```python
from build123d import *

# Parameters (mm, degrees)
SKETCH1_W                                       = 100
SKETCH1_H                                       = 55
BOSS_EXTRUDE1_DEPTH                             = 5
SKETCH2_W                                       = 5
SKETCH2_H                                       = 55
BOSS_EXTRUDE2_DEPTH                             = 15
CUT_EXTRUDE1_REACH                              = 22
CSK_FOR_M2_FLAT_HEAD_MACHINE_SCREW1_D           = 2.4
CSK_FOR_M2_FLAT_HEAD_MACHINE_SCREW1_CSINK_D     = 4.4
CSK_FOR_M2_FLAT_HEAD_MACHINE_SCREW1_CSINK_ANGLE = 90
CUT_EXTRUDE2_REACH                              = 22
SKETCH6_R                                       = 4


with BuildPart() as part:
    # Sketch1 → Boss-Extrude1 (new body)
    with BuildSketch(Plane(origin=(0, 0, 0), x_dir=(0, 0, -1), z_dir=(1, 0, 0))):
        Rectangle(SKETCH1_W, SKETCH1_H)
    extrude(amount=BOSS_EXTRUDE1_DEPTH)

    # Sketch2 → Boss-Extrude2 (add)
    with BuildSketch(Plane(origin=(5, 0, 0), x_dir=(0, 0, -1), z_dir=(1, 0, 0))):
        with Locations((47.5, 0)):
            Rectangle(SKETCH2_W, SKETCH2_H)
    extrude(amount=BOSS_EXTRUDE2_DEPTH)

    # Sketch3 → Cut-Extrude1 (cut, up to next)
    with BuildSketch(Plane.ZY, mode=Mode.PRIVATE) as cut_extrude1_sk1:
        Polygon((50, 27.5), (40, 27.5), (50, 17.5), align=None)
    cut_extrude1_tool1 = extrude(cut_extrude1_sk1.sketch, amount=-CUT_EXTRUDE1_REACH, mode=Mode.PRIVATE) & part.part
    add(cut_extrude1_tool1.solids().sort_by_distance((0, 24.166667, 46.666667))[0], mode=Mode.SUBTRACT)
    # Sketch3 → Cut-Extrude1 (cut, up to next)
    with BuildSketch(Plane.ZY, mode=Mode.PRIVATE) as cut_extrude1_sk2:
        Polygon((50, -27.5), (40, -27.5), (50, -17.5), align=None)
    cut_extrude1_tool2 = extrude(cut_extrude1_sk2.sketch, amount=-CUT_EXTRUDE1_REACH, mode=Mode.PRIVATE) & part.part
    add(cut_extrude1_tool2.solids().sort_by_distance((0, -24.166667, 46.666667))[0], mode=Mode.SUBTRACT)

    # CSK for M2 Flat Head Machine Screw1 (through all)
    with Locations(Plane.XY.offset(-45)):
        with Locations((12.5, 15.5), (12.5, -15.5)):
            CounterSinkHole(CSK_FOR_M2_FLAT_HEAD_MACHINE_SCREW1_D / 2, CSK_FOR_M2_FLAT_HEAD_MACHINE_SCREW1_CSINK_D / 2, counter_sink_angle=CSK_FOR_M2_FLAT_HEAD_MACHINE_SCREW1_CSINK_ANGLE)

    # Sketch6 → Cut-Extrude2 (cut, up to next)
    with BuildSketch(Plane.ZY, mode=Mode.PRIVATE) as cut_extrude2_sk1:
        with Locations((22.5, 0)):
            Circle(SKETCH6_R)
    cut_extrude2_tool1 = extrude(cut_extrude2_sk1.sketch, amount=-CUT_EXTRUDE2_REACH, mode=Mode.PRIVATE) & part.part
    add(cut_extrude2_tool1.solids().sort_by_distance((0, 0, 22.5))[0], mode=Mode.SUBTRACT)


solid = part.part
```
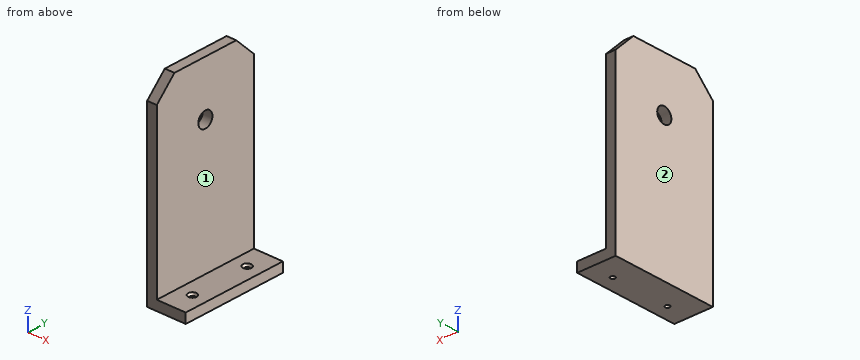
Geometry check sheet. Reference: the model listing, model coordinates, mm. Face numbers are marked on the shaded views. A direction names the side the tool comes from. Coordinates: 2 decimals unless noted, no trailing zeros. Order: outer loops, then holes, each group sorted by start corner. A loop starts at its lowest first (then second) coordinate and runs counter-clockwise, first axis right, second up.
Q1. Sectioned sample at C-C on z = 22.5. Record the cut outline in (x, y).
Reply:
outline: (0, -27.5) - (5, -27.5) - (5, -4) - (0, -4) - close; (0, 4) - (5, 4) - (5, 27.5) - (0, 27.5) - close
Q2. Sectioned sample at B-B on x = 12.5. Record the cut outline in (y, z), and give its area (3 significant figures).
Reply:
outline: (-27.5, -50) - (-16.7, -50) - (-16.7, -46) - (-17.7, -45) - (-27.5, -45) - close; (-14.3, -50) - (14.3, -50) - (14.3, -46) - (13.3, -45) - (-13.3, -45) - (-14.3, -46) - close; (16.7, -50) - (27.5, -50) - (27.5, -45) - (17.7, -45) - (16.7, -46) - close
area: 249 mm2
Q3. Thickness scan on probe 1 along Y at (x, z) = (12.5, -47); probe 2 along X at (y, z) = (-16, 9.5); probe 3 along Z at (x, y) = (14, -23.5). Record the ranges inside material, lowest first.
Reply:
probe 1: y = -27.5 to -16.7, -14.3 to 14.3, 16.7 to 27.5
probe 2: x = 0 to 5
probe 3: z = -50 to -45
Q4. Depth check by flat-ended pin: pin 1 Ø8 at (y, z) = (6.5, -25) entering from +X; pin 2 Ø6.5 at (y, z) = (0, 22.5) entering from +X; pin 3 Ø3 at (x, y) = (12.5, 15.5) entering from +Z; pin 4 Ø2 at (x, y) = (11, -12) entering from +Z. Enter the tip coordinate at first touch or a pass-through.
Reply:
pin 1: stops at x = 5
pin 2: passes through
pin 3: stops at z = -45.7
pin 4: stops at z = -45
Q5. Sectioned sample at D-D on y = -8.5. Record the cut outline in (x, z), and give its area (3 significant figures).
Reply:
outline: (0, -50) - (20, -50) - (20, -45) - (5, -45) - (5, 50) - (0, 50) - close
area: 575 mm2
Q6. Sectioned sample at A-A on y = -15.5. Record the cut outline in (x, z), and give its area (3 significant figures).
Reply:
outline: (0, -50) - (11.3, -50) - (11.3, -46) - (10.3, -45) - (5, -45) - (5, 50) - (0, 50) - close; (13.7, -50) - (20, -50) - (20, -45) - (14.7, -45) - (13.7, -46) - close
area: 562 mm2
Q7. Tool access check on the marked faces 1 and 2. Record the directions out of +Z, -Z, +X, -X, +Y, -Y that give a thin tool (end or side, any length) a straight path to the whole face; none if there is none.
Reply:
face 1: +Z, +X, +Y, -Y
face 2: +Z, -Z, -X, +Y, -Y
